Autodesk Fusion 360 part; units mm, degrees
sketch "Sketch1" plane through (0, 0, 0) normal (0, 0, 1) x (1, 0, 0)
  line L0 (-100, 90) -> (0, 90)
  line L1 (0, 90) -> (0, -80)
  line L2 (0, -80) -> (-100, -80)
  line L3 (-100, -80) -> (-100, 90)
  line L4 (0, 90) -> (90, 90)
  line L5 (90, 90) -> (90, 0)
  line L6 (90, 0) -> (0, 0)
  line L7 (0, 0) -> (0, 90)
  dimension "d1" = 100
  dimension "d2" = 170
  dimension "d3" = 90
  dimension "d4" = 90
extrude "Extrude1" add sketch "Sketch1" along normal blind 3
sketch "Sketch2" plane through (0, 0, 3) normal (0, 0, 1) x (-1, 0, 0)
  line L0 (-90, 0) -> (-90, -90)
  line L1 (-90, -90) -> (100, -90)
  line L2 (100, -90) -> (100, 80)
  line L3 (100, 80) -> (0, 80)
  line L4 (0, 80) -> (0, 0)
  line L5 (0, 0) -> (-90, 0)
  line L6 (97, -87) -> (3, -87)
  line L7 (3, -87) -> (3, 77)
  line L8 (3, 77) -> (97, 77)
  line L9 (97, 77) -> (97, -87)
  line L10 (3, -87) -> (-87, -87)
  line L11 (-87, -87) -> (-87, -3)
  line L12 (-87, -3) -> (3, -3)
  line L13 (3, -3) -> (3, -87)
  dimension "d7" = 3
  dimension "d8" = 3
  dimension "d9" = 3
  dimension "d10" = 3
  dimension "d12" = 97
  dimension "d13" = 3
extrude "Extrude2" add sketch "Sketch2" along normal blind 40
sketch "Sketch3" plane through (0, 0, 3) normal (0, 0, 1) x (-1, 0, 0)
  line L0 (-87, -87) -> (97, -87)
  line L1 (97, -87) -> (97, 77)
  line L2 (97, 77) -> (3, 77)
  line L3 (3, 77) -> (3, -3)
  line L4 (3, -3) -> (-87, -3)
  line L5 (-87, -3) -> (-87, -87)
  circle A0 centre (-45, -45) radius 15
  line L6 (-90, -90) -> (100, -90)
  line L7 (-90, 0) -> (-90, -90)
  dimension "d16" = 30
  dimension "d17" = 45
  dimension "d18" = 45
extrude "Extrude3" add sketch "Sketch3" along normal blind 30 contours A0
sketch "Sketch4" plane through (0, 0, 33) normal (0, 0, 1) x (-1, 0, 0)
  circle A0 centre (-45, -45) radius 15
  circle A1 centre (-45, -45) radius 2
  dimension "d21" = 4
extrude "Extrude4" cut sketch "Sketch4" against normal blind 30 contours A1
fillet "Fillet1" radius 2 1 edges at (58.9849, 50.4242, 33)
sketch "Sketch5" plane through (-97, 0, 0) normal (1, 0, 0) x (0, 1, 0)
  line L0 (-77, 3) -> (87, 3)
  line L1 (87, 3) -> (87, 43)
  line L2 (87, 43) -> (-77, 43)
  line L3 (-77, 43) -> (-77, 3)
  line L4 (87, 43) -> (83, 43)
  line L5 (83, 43) -> (83, 36)
  line L6 (83, 36) -> (87, 36)
  line L7 (87, 36) -> (87, 43)
  dimension "d26" = 4
  dimension "d27" = 7
extrude "Extrude5" add sketch "Sketch5" along normal blind 4 contours L1 L2 L4 L5 L6 L7
sketch "Sketch6" plane through (0, 0, 43) normal (0, 0, 1) x (-1, 0, 0)
  line L0 (-87, -87) -> (-87, -3)
  line L1 (-87, -3) -> (3, -3)
  line L2 (3, -3) -> (3, 77)
  line L3 (3, 77) -> (97, 77)
  line L4 (97, 77) -> (97, -83)
  line L5 (97, -83) -> (93, -83)
  line L6 (93, -83) -> (93, -87)
  line L7 (93, -87) -> (-87, -87)
  line L8 (0, 0) -> (-90, 0)
  line L9 (-90, 0) -> (-90, -90)
  line L10 (-90, -90) -> (100, -90)
  line L11 (100, -90) -> (100, 80)
  line L12 (100, 80) -> (0, 80)
  line L13 (0, 80) -> (0, 0)
  line L14 (3, 77) -> (7, 77)
  line L15 (7, 77) -> (7, 73)
  line L16 (7, 73) -> (3, 73)
  line L17 (3, 73) -> (3, 77)
  line L18 (97, 77) -> (93, 77)
  line L19 (93, 77) -> (93, 73)
  line L20 (93, 73) -> (97, 73)
  line L21 (97, 73) -> (97, 77)
  line L22 (-87, -87) -> (-83, -87)
  line L23 (-83, -87) -> (-83, -83)
  line L24 (-83, -83) -> (-87, -83)
  line L25 (-87, -83) -> (-87, -87)
  line L26 (-87, -3) -> (-83, -3)
  line L27 (-83, -3) -> (-83, -7)
  line L28 (-83, -7) -> (-87, -7)
  line L29 (-87, -7) -> (-87, -3)
  circle A0 centre (-85, -5) radius 1.1
  circle A1 centre (-85, -85) radius 1.1
  circle A2 centre (5, 75) radius 1.1
  circle A3 centre (95, 75) radius 1.1
  dimension "d30" = 4
  dimension "d31" = 4
  dimension "d32" = 4
  dimension "d33" = 4
  dimension "d34" = 4
  dimension "d35" = 4
  dimension "d36" = 4
  dimension "d37" = 4
  dimension "d38" = 2.2
  dimension "d39" = 2
  dimension "d40" = 2
  dimension "d41" = 2.2
  dimension "d42" = 2
  dimension "d43" = 2
  dimension "d44" = 2.2
  dimension "d45" = 2
  dimension "d46" = 2
  dimension "d47" = 2.2
  dimension "d48" = 2
  dimension "d49" = 2
extrude "Extrude6" add sketch "Sketch6" against normal blind 7 contours L0 L7 L22 L23 L24 L25 | L0 L1 L26 L27 L28 L29 | L3 L4 L18 L19 L20 L21 | L2 L3 L14 L15 L16 L17
sketch "Sketch7" plane through (0, 0, 43) normal (0, 0, 1) x (-1, 0, 0)
  circle A0 centre (-85, -85) radius 1.1
  circle A1 centre (5, 75) radius 1.1
  circle A2 centre (-85, -5) radius 1.1
  circle A3 centre (95, 75) radius 1.1
  line L0 (-87, -83) -> (-87, -7)
  line L1 (-87, -7) -> (-83, -7)
  line L2 (-83, -7) -> (-83, -3)
  line L3 (-83, -3) -> (3, -3)
  line L4 (3, -3) -> (3, 73)
  line L5 (3, 73) -> (7, 73)
  line L6 (7, 73) -> (7, 77)
  line L7 (7, 77) -> (93, 77)
  line L8 (93, 77) -> (93, 73)
  line L9 (93, 73) -> (97, 73)
  line L10 (97, 73) -> (97, -83)
  line L11 (97, -83) -> (93, -83)
  line L12 (93, -83) -> (93, -87)
  line L13 (93, -87) -> (-83, -87)
  line L14 (-83, -87) -> (-83, -83)
  line L15 (-83, -83) -> (-87, -83)
  line L16 (0, 0) -> (-90, 0)
  line L17 (-90, 0) -> (-90, -90)
  line L18 (-90, -90) -> (100, -90)
  line L19 (100, -90) -> (100, 80)
  line L20 (100, 80) -> (0, 80)
  line L21 (0, 80) -> (0, 0)
  circle A4 centre (95, -85) radius 1.1
  dimension "d52" = 2.2
  dimension "d53" = 2
  dimension "d54" = 2
extrude "Extrude7" cut sketch "Sketch7" against normal blind 7 contours A4
sketch "Sketch8" plane through (0, 90, 0) normal (0, 1, 0) x (-1, 0, 0)
  line L0 (-90, 0) -> (100, 0)
  line L1 (100, 0) -> (100, 43)
  line L2 (100, 43) -> (-90, 43)
  line L3 (-90, 43) -> (-90, 0)
  line L4 (-3, 37) -> (45, 37)
  line L5 (45, 37) -> (45, 9)
  line L6 (45, 9) -> (-3, 9)
  line L7 (-3, 9) -> (-3, 37)
  dimension "d57" = 48
  dimension "d58" = 28
  dimension "d59" = 55
  dimension "d60" = 6
extrude "Extrude8" cut sketch "Sketch8" against normal blind 3 contours L4 L5 L6 L7
sketch "Sketch9" plane through (0, 0, 3) normal (0, 0, 1) x (-1, 0, 0)
  circle A0 centre (-45, -45) radius 15
  line L0 (-87, -87) -> (97, -87)
  line L1 (97, -87) -> (97, 77)
  line L2 (97, 77) -> (3, 77)
  line L3 (3, 77) -> (3, -3)
  line L4 (3, -3) -> (-87, -3)
  line L5 (-87, -3) -> (-87, -87)
  line L6 (21, 71) -> (91, 71)
  line L7 (91, 71) -> (91, -43)
  line L8 (91, -43) -> (21, -43)
  line L9 (21, -43) -> (21, 71)
  circle A1 centre (21, 71) radius 4
  circle A2 centre (91, 71) radius 4
  circle A3 centre (21, -43) radius 4
  circle A4 centre (91, -43) radius 4
  circle A5 centre (91, -43) radius 1.9
  circle A6 centre (21, -43) radius 1.9
  circle A7 centre (91, 71) radius 1.9
  circle A8 centre (21, 71) radius 1.9
  dimension "d63" = 70
  dimension "d64" = 114
  dimension "d65" = 6
  dimension "d66" = 6
  dimension "d67" = 8
  dimension "d68" = 8
  dimension "d69" = 8
  dimension "d70" = 8
  dimension "d79" = 3.8
  dimension "d80" = 3.8
  dimension "d81" = 3.8
  dimension "d82" = 3.8
extrude "Extrude9" add sketch "Sketch9" along normal blind 5 contours L6 L9 A8 | L6 L9 A8 | L6 L9 A1 A8 | L6 L9 A1 A8 | L6 L7 A2 A7 | L6 L7 A2 A7 | L8 L9 A3 A6 | L8 L9 A3 A6 | L6 L7 A7 | L6 L7 A7 | L8 L9 A6 | L8 L9 A6 | L7 L8 A4 A5 | L7 L8 A4 A5 | L7 L8 A5 | L7 L8 A5
sketch "Sketch10" plane through (0, 0, 8) normal (0, 0, 1) x (-1, 0, 0)
  circle A0 centre (21, 71) radius 4
  circle A1 centre (21, 71) radius 1.8
  circle A2 centre (91, 51) radius 1.8
  circle A3 centre (91, -63) radius 1.8
  circle A4 centre (27, -63) radius 1.8
  dimension "d73" = 3.6
  dimension "d74" = 3.6
  dimension "d75" = 3.6
  dimension "d76" = 3.6
extrude "Extrude10" cut sketch "Sketch10" against normal blind 5 contours A1 | A2 | A3 | A4
sketch "Sketch11" plane through (0, 0, 8) normal (0, 0, 1) x (-1, 0, 0)
  circle A0 centre (21, -43) radius 4
  circle A1 centre (21, -43) radius 1.9
  circle A2 centre (91, -43) radius 1.9
  circle A3 centre (91, -43) radius 4
  circle A4 centre (91, 71) radius 1.9
  circle A5 centre (91, 71) radius 4
  dimension "d83" = 3.8
  dimension "d84" = 3.8
  dimension "d85" = 3.8
extrude "Extrude11" cut sketch "Sketch11" against normal blind 5 contours A1 | A2 | A4
sketch "Sketch12" plane through (0, 90, 0) normal (0, 1, 0) x (-1, 0, 0)
  line L0 (45, 37) -> (45, 9)
  line L1 (45, 9) -> (-3, 9)
  line L2 (-3, 9) -> (-3, 37)
  line L3 (-3, 37) -> (45, 37)
  line L4 (-90, 0) -> (100, 0)
  line L5 (100, 0) -> (100, 43)
  line L6 (100, 43) -> (-90, 43)
  line L7 (-90, 43) -> (-90, 0)
  circle A0 centre (75, 25) radius 3
  dimension "d88" = 6
extrude "Extrude12" cut sketch "Sketch12" against normal blind 3 contours A0
Could you check a few things on this model? Use its own coordinates, in mm. A direction names the side the tool comes from. Round coordinates to 2 decimals unless told otherwise and drop trailing zeros. Loops run counter-clockwise (first coordinate to the right, second up) from the corner with the lowest first, then second, coordinate; pieces in that order, holes last.
Q1. I want a section at A-A (z = 16.5). Write out the boundary of the cut face in (x, y), and give its area (3 significant figures).
Q2. Thinking about a two-plate mould opening in Y: for faces 4 (the flat face through (-5.4, 87.2, 43)), 5 (the flat face through (87, 46, 23)), which applies, pulls with the +Y half, pulls with the -Y half, needs draft (parallel to the pull), parting line crosses it, or undercut?
Q3. I want a section at C-C (y = -37). Write out the boundary of the cut face in (x, z).
Q4. I want a section at B-B (z = 5.5). Give the number of separate pieces and of enclosed holes in the cut face, and give its area (3 significant figures).
Q5. On a 3-axis mill with a long thin cutter (end or side, diameter ignored), from which of +Z, -Z, +X, -X, +Y, -Y can I reach the whole of each face in a straight line? I mean faces 1 (the flat face through (-93, -75, 40)), 2 (the flat face through (0, -41, 21)), 3 (the flat face through (84, 4, 36)). Say none if no direction works.
Q6. Please list where these lines run through material, in increasing order: L1, parallel to X at y = -75, z = 41; L2, parallel to X at y = 45, z = 19.25; L3, parallel to Y at x = 85, z = 38.5.
Q7. For P1, Ø2.5, axis at x = -95, y = -75, coming from the +Z side; P2, Ø6, axis at x = -21, y = -71, coming from the +Z side; P3, Ø10, axis at x = 32, z = 38.5, coming from the -Y side; P4, Ø8, axis at x = 48, y = 50, coming from the +Z side, each with a flat end and sliding along its axis, tell me the tip position at first contact or that it passes through.
Answer below:
1. outline: (-100, -80) - (0, -80) - (0, 0) - (90, 0) - (90, 90) - (3, 90) - (3, 87) - (87, 87) - (87, 3) - (-3, 3) - (-3, -77) - (-97, -77) - (-97, 87) - (-45, 87) - (-45, 90) - (-100, 90) - close; circle Ø30 at (45, 45); hole circle Ø4 at (45, 45)
1. area: 2,670 mm2
2. face 4: needs draft
2. face 5: undercut
3. outline: (-100, 0) - (0, 0) - (0, 43) - (-3, 43) - (-3, 3) - (-97, 3) - (-97, 43) - (-100, 43) - close
4. separate pieces: 6
4. enclosed holes: 6
4. area: 2,980 mm2
5. face 1: +Z
5. face 2: +Z, -Z, +X, -Y
5. face 3: none
6. L1: x = -100 to -96.1, -93.9 to -93, -7 to -6.1, -3.9 to 0
6. L2: x = -100 to -97, 30 to 43, 47 to 60, 87 to 90
6. L3: y = 0 to 3.9, 6.1 to 7, 83 to 83.9, 86.1 to 90
7. P1: stops at z = 43
7. P2: stops at z = 8
7. P3: stops at y = 0
7. P4: stops at z = 33
